The listing builds one solid part. Answer for the finished solid, in the listing's coordinates (mm). Face numbers are marked on the shaded views. A direction names the side the tool comes from. Round coordinates to 2 decimals unless told otherwise and drop trailing zeros. Write each loop counter-clockwise with the first axis right and the second up, starting at its lowest first coordinate (ties: lowest second). Pieces come first, ordered by that corner, then holes. Notation, with made-up numbers: (37, 43) - (55, 43) arc R20 ccw to (55, 65) - close; hole circle Ø1 at (53.5, 41.5). An arc over 180 degrees is marked (long way). Answer in a Markdown table with one row per item.
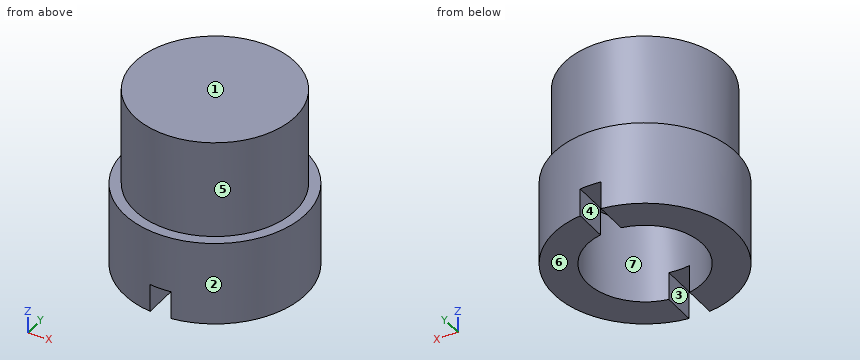
from build123d import *

# Parameters (mm, degrees)
SKETCH1_R               = 10.3124
SKETCH1_R_2             = 6.5405
BOSS_EXTRUDE1_DEPTH     = 9.525
SKETCH2_R               = 9.1186
BOSS_EXTRUDE2_DEPTH     = 11.0998
CUT_EXTRUDE1_DEPTH      = 19.327486122
CUT_EXTRUDE1_DEPTH_BACK = 19.327486122
SKETCH3_W               = 2.3622
SKETCH3_H               = 3.175


with BuildPart() as part:
    # Sketch1 → Boss-Extrude1 (new body)
    with BuildSketch(Plane.XY):
        Circle(SKETCH1_R)
        Circle(SKETCH1_R_2, mode=Mode.SUBTRACT)
    extrude(amount=-BOSS_EXTRUDE1_DEPTH)

    # Sketch2 → Boss-Extrude2 (add)
    with BuildSketch(Plane.XY):
        Circle(SKETCH2_R)
    extrude(amount=BOSS_EXTRUDE2_DEPTH)

    # Sketch3 → Cut-Extrude1 (cut, two sides: drawn at the far end of the back side and taken through both)
    with BuildSketch(Plane(origin=(0, 0, 0), x_dir=(1, 0, 0), z_dir=(0, 1, 0)).offset(-CUT_EXTRUDE1_DEPTH_BACK)):
        with Locations((0, 7.9375)):
            Rectangle(SKETCH3_W, SKETCH3_H)
    extrude(amount=CUT_EXTRUDE1_DEPTH + CUT_EXTRUDE1_DEPTH_BACK, mode=Mode.SUBTRACT)


solid = part.part
(1) Section C-C (z = 1.5) is taken. Give the vertices of the cut face in (x, y).
Checked values:
| item | result |
|---|---|
| outline | circle Ø18.24 at (0, 0) |
(2) Section D-D (z = -4.25) is taken. Give the vertices of the cut face in (x, y).
Checked values:
| item | result |
|---|---|
| outline | circle Ø20.62 at (0, 0); hole circle Ø13.08 at (0, 0) |
(3) Section A-A (y = 0) is taken. Give the vertices of the cut face in (x, z) (1 decimal).
Checked values:
| item | result |
|---|---|
| outline | (-10.3, -9.5) - (-6.5, -9.5) - (-6.5, 0) - (6.5, 0) - (6.5, -9.5) - (10.3, -9.5) - (10.3, 0) - (9.1, 0) - (9.1, 11.1) - (-9.1, 11.1) - (-9.1, 0) - (-10.3, 0) - close |
(4) Find the intervals of material crossed by line 1 (Y direction, x = 0, z = -2.25); line 2 (Z direction, x = -0.5, y = 7.25); line 3 (Y direction, x = 3, z = -3), in increasing order.
Checked values:
| item | result |
|---|---|
| line 1 | y = -10.31 to -6.54, 6.54 to 10.31 |
| line 2 | z = -6.35 to 11.1 |
| line 3 | y = -9.87 to -5.81, 5.81 to 9.87 |
(5) For a pull along X with two mould halves and no side action, classify the marked faces 1, 2, 3 and 4 as pulls with the +X half, pulls with the -X half, needs draft (parallel to the pull), parting line crosses it, or undercut.
Checked values:
| item | result |
|---|---|
| face 1 | needs draft |
| face 2 | parting line crosses it |
| face 3 | undercut |
| face 4 | undercut |
(6) For the marked faces 5, 6 and 7, determine the directions among +Z, -Z, +X, -X, +Y, -Y from which every point of the face is accessible in a straight line to the end or side of a thin tool.
Checked values:
| item | result |
|---|---|
| face 5 | +Z |
| face 6 | -Z, +X, -X, +Y, -Y |
| face 7 | -Z |
(7) Flat-ended cylindrical pins translate along their axes: pin 1 (3 mm diameter, centred on x = -0.5, y = 2, fed in from -Z); pin 2 (3.5 mm diameter, centred on y = -8.5, z = -8, fed in from -X); pin 3 (2 mm diameter, centred on x = -6, z = -1.5, fed in from -Y). Find the tip coordinate at first contact, or state that the pin passes through.
Checked values:
| item | result |
|---|---|
| pin 1 | stops at z = 0 |
| pin 2 | stops at x = -7.8 |
| pin 3 | stops at y = -9.02 |
(8) Section B-B (x = 0) is taken. Give the vertices of the cut face in (y, z), and give its area (3 significant figures).
Checked values:
| item | result |
|---|---|
| outline | (-10.31, -6.35) - (-6.54, -6.35) - (-6.54, 0) - (6.54, 0) - (6.54, -6.35) - (10.31, -6.35) - (10.31, 0) - (9.12, 0) - (9.12, 11.1) - (-9.12, 11.1) - (-9.12, 0) - (-10.31, 0) - close |
| area | 250 mm2 |
